```python
from build123d import *

# Parameters (mm, degrees)
SKETCH_1_W                = 105
SKETCH_1_H                = 80
SKETCH_1_R                = 2.5
SKETCH_1_W_2              = 5
SKETCH_1_H_2              = 15
EXTRUDE_1_DEPTH           = 5
HOLE_WIZARD_1_D           = 5.5
HOLE_WIZARD_1_CBORE_D     = 10
HOLE_WIZARD_1_CBORE_DEPTH = 5.7
SKETCH_4_R                = 2.75
CUT_EXTRUDE_1_DEPTH       = 84.779472426


with BuildPart() as part:
    # 草图1 → 凸台-拉伸1 (new, symmetric)
    # profile 1 of 3: a face of its own
    with BuildSketch(Plane.XY):
        Rectangle(SKETCH_1_W, SKETCH_1_H)
        with Locations((42.5, 25)):
            Circle(SKETCH_1_R, mode=Mode.SUBTRACT)
        with Locations((-42.5, 25)):
            Circle(SKETCH_1_R, mode=Mode.SUBTRACT)
        with Locations((42.5, -25)):
            Circle(SKETCH_1_R, mode=Mode.SUBTRACT)
        with Locations((-42.5, -25)):
            Circle(SKETCH_1_R, mode=Mode.SUBTRACT)
    # profile 2 of 3: a face of its own
    with BuildSketch(Plane.XY):
        with Locations((-8, 47.5)):
            Rectangle(SKETCH_1_W_2, SKETCH_1_H_2)
    # profile 3 of 3: a face of its own
    with BuildSketch(Plane.XY):
        with Locations((8, 47.5)):
            Rectangle(SKETCH_1_W_2, SKETCH_1_H_2)
    extrude(amount=EXTRUDE_1_DEPTH, both=True)

    # 打孔尺寸(%根据)内六角圆柱头螺钉的类型1 (through all)
    with Locations(Plane.XY.offset(5)):
        with Locations((-42.5, 25), (42.5, 25), (42.5, -25), (-42.5, -25)):
            CounterBoreHole(HOLE_WIZARD_1_D / 2, HOLE_WIZARD_1_CBORE_D / 2, HOLE_WIZARD_1_CBORE_DEPTH)

    # 草图4 → 切除-拉伸1 (cut, through all)
    with BuildSketch(Plane.ZY.offset(10.5)):
        with Locations(Location((0, 50, 0), (0, 0, 270))):
            Circle(SKETCH_4_R)
    extrude(amount=-CUT_EXTRUDE_1_DEPTH, mode=Mode.SUBTRACT)


solid = part.part
```
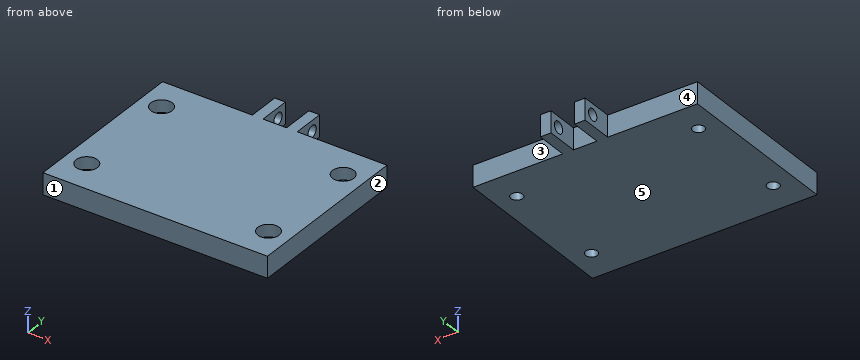
Input: part model. Units: mm. Frame: model coordinates. Face numbers are marked on the shaded views. A direction names the side the tool comes from. Give positions to 0.01 mm unless a question says otherwise; leave off trailing zeros. Order: outer loops, then holes, each group sorted by start corner. A loop starts at its lowest first (then second) coordinate and runs counter-clockwise, first axis right, second up. Notation, with made-up numbers: M 57.25,47.25 L 87.25,47.25 A16 ccw 87.25,64.25 Z; hole C 54,-15 d8. An arc over 180 degrees is marked long. Return JSON: item names as keys, results as strings.
Item 1: First-contact query: P1, Ø4.5, axis at y = 50, z = 0, coming from the +X side; P2, Ø3, axis at x = 40.5, y = 24.5, coming from the +Z side; P3, Ø3, axis at y = 47.5, z = 1, coming from the +X side; P4, Ø5, axis at y = 44.5, z = -0.5, coming from the -X side. Flat tips, straight axial feed; report the tip coordinate or a pass-through.
Solutions:
{"P1": "through", "P2": "z = -0.7", "P3": "x = 10.5", "P4": "x = -10.5"}
Item 2: Access query for the marked faces 4 and 5. Directions: +Z, -Z, +X, -X, +Y, -Y. A direction counts if a zero-diameter tool reaches every point of the face in a straight line with its end or side. Return the directions, or none.
Solutions:
{"face 4": "+Z, -Z, -X, +Y", "face 5": "-Z, +X, -X, +Y, -Y"}
Item 3: Ray query, probe 1 along Y at (x, z) = (42.5, -3.5); probe 2 along Y at (x, z) = (-42.5, 1.4); probe 3 along X at (y, z) = (23.5, -3.75). Return the intervals inside material, ascending.
Solutions:
{"probe 1": "-40 to -27.75, -22.25 to 22.25, 27.75 to 40", "probe 2": "-40 to -30, -20 to 20, 30 to 40", "probe 3": "-52.5 to -44.8, -40.2 to 40.2, 44.8 to 52.5"}
Item 4: Cut plane A-A (z = 1.5). Return loops of the section in (x, y).
Solutions:
{"outline": "M -52.5,-40 L 52.5,-40 L 52.5,40 L 10.5,40 L 10.5,47.7 L 5.5,47.7 L 5.5,40 L -5.5,40 L -5.5,47.7 L -10.5,47.7 L -10.5,40 L -52.5,40 Z; M -10.5,52.3 L -5.5,52.3 L -5.5,55 L -10.5,55 Z; M 5.5,52.3 L 10.5,52.3 L 10.5,55 L 5.5,55 Z; hole C -42.5,-25 d10; hole C -42.5,25 d10; hole C 42.5,-25 d10; hole C 42.5,25 d10"}
Item 5: Cut plane C-C (x = 42.5). Return loops of the section in (y, z).
Solutions:
{"outline": "M -40,-5 L -27.75,-5 L -27.75,-0.7 L -30,-0.7 L -30,5 L -40,5 Z; M -22.25,-5 L 22.25,-5 L 22.25,-0.7 L 20,-0.7 L 20,5 L -20,5 L -20,-0.7 L -22.25,-0.7 Z; M 27.75,-5 L 40,-5 L 40,5 L 30,5 L 30,-0.7 L 27.75,-0.7 Z"}
Item 6: Cut plane B-B (y = 44). Return loops of the section in (x, z).
Solutions:
{"outline": "M -10.5,-5 L -5.5,-5 L -5.5,5 L -10.5,5 Z; M 5.5,-5 L 10.5,-5 L 10.5,5 L 5.5,5 Z"}
Item 7: Pull-direction query (Y, two-part tool) for the marked faces 1, 2 and 3; classes: +Y half, -Y half, draft (parallel to the pull), parting line (faces both ways), or undercut.
Solutions:
{"face 1": "-Y half", "face 2": "draft", "face 3": "+Y half"}
Item 8: Cut plane D-D (y = 25). Return loops of the section in (x, z), then the cut area to 3 significant figures.
Solutions:
{"outline": "M -52.5,-5 L -45.25,-5 L -45.25,-0.7 L -47.5,-0.7 L -47.5,5 L -52.5,5 Z; M -39.75,-5 L 39.75,-5 L 39.75,-0.7 L 37.5,-0.7 L 37.5,5 L -37.5,5 L -37.5,-0.7 L -39.75,-0.7 Z; M 45.25,-5 L 52.5,-5 L 52.5,5 L 47.5,5 L 47.5,-0.7 L 45.25,-0.7 Z", "area": "889 mm^2"}
